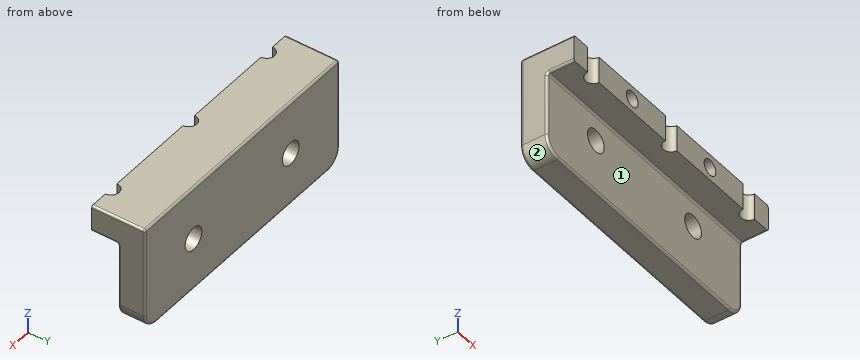
```python
from build123d import *

# Parameters (mm, degrees)
F0_W     = 50
F0_H     = 15
F1_DEPTH = 5
F2_D     = 4.3
F0_H_2   = 5
F3_DEPTH = 10
F5_D     = 2.95
F6_R     = 3
F7_R     = 0.4
F9_D     = 3
F9_DEPTH = 6
F9_TIP   = 0.9012909285


with BuildPart() as f1:
    # F0 (on Front) → F1 (new body)
    with BuildSketch(Plane.XZ):
        with Locations((0, -2.5)):
            Rectangle(F0_W, F0_H)
    extrude(amount=F1_DEPTH)

    # F2 (through all)
    with Locations(Plane(origin=(0, 0, 0), x_dir=(1, 0, 0), z_dir=(0, 1, 0))):
        with Locations((12.5, 0), (-12.5, 0)):
            Hole(F2_D / 2)

    # F0 (on Front) → F3 (join)
    with BuildSketch(Plane.XZ):
        with Locations((0, 7.5)):
            Rectangle(F0_W, F0_H_2)
    extrude(amount=F3_DEPTH)

    # F5 (through all)
    with Locations(Plane.XY.offset(10)):
        with Locations((-20, -10), (0, -10), (20, -10)):
            Hole(F5_D / 2)

    # F6
    f6_edges = [f1.edges().sort_by_distance(p)[0] for p in [
        (-25, -2.5, -10),
        (25, -2.5, -10),
    ]]
    fillet(f6_edges, radius=F6_R)

    # F7
    f7_edges = [f1.edges().sort_by_distance(p)[0] for p in [
        (0, 0, 10),
        (-25, 0, 1.5),
        (-25, -5, 10),
        (25, -5, 10),
        (0, -5, -10),
        (0, -5, 5),
        (25, -5, -1),
        (25, -7.5, 5),
        (25, 0, 1.5),
        (24.12132, -5, -9.12132),
        (-25, -5, -1),
        (-24.12132, -5, -9.12132),
        (24.12132, 0, -9.12132),
        (-25, -7.5, 5),
        (0, 0, -10),
        (-24.12132, 0, -9.12132),
    ]]
    fillet(f7_edges, radius=F7_R)

    # F9
    with Locations(Plane.XZ.offset(10)):
        with Locations((-10, 7.5), (10, 7.4705528095)):
            Hole(F9_D / 2, depth=F9_DEPTH)
            with Locations((0, 0, -(F9_DEPTH + F9_TIP / 2))):  # 118° drill point
                Cone(0, F9_D / 2, F9_TIP, mode=Mode.SUBTRACT)


solid = f1.part
```
Verification items for the finished model (mm, model axes). Face numbers are marked on the shaded views. A direction names the side the tool comes from. Coordinates: 2 decimals unless noted, no trailing zeros. Write each loop counter-clockwise with the first axis right and the second up, starting at its lowest first coordinate (ties: lowest second). Pieces come first, ordered by that corner, then holes. Notation, with made-up numbers: M 65,75.25 L 76,75.25 A30 ccw 76,105.25 Z; hole C 6,16.25 d9. An arc over 180 degrees is marked long. Answer as a JSON object with one key per item and string values. Group by question number.
(1) Cross-section at C-C, the plane y = -9.5. Record the cut outline in (x, z).
(2) Material ranges on line 1 (X direction, y = -6.4, z = 7.5); line 2 (Z direction, x = 10, y = -7.95); line 3 (Z direction, x = -12.5, y = -0.95), recorded low to high.
(3) Cross-section at D-D, the plane x = 0. Record the cut outline in (y, z) (3 decimals).
(4) Cross-section at B-B, the plane z = 0. Record the cut outline in (x, y), and give its area (3 significant figures).
(5) Tool access check on the marked faces 1 and 2. Record the directions out of +Z, -Z, +X, -X, +Y, -Y that give a thin tool (end or side, any length) a straight path to the whole face; none if there is none.
(6) Gauge pin test, flat ends, axial feed: pin 1 (3.5 mm diameter, centred on x = 12.5, z = 0, fed in from +Y) (1 decimal); pin 2 (5 mm diameter, centred on x = -1, y = -7, fed in from -Z). Record the tip position at first contact, or that the pin passes through.
(7) Cross-section at A-A, the plane x = 12.5. Record the cut outline in (y, z).
Reply:
{
 "1": {"outline": "M -25,5.4 A0.4 ccw -24.6,5 L -21.39,5 L -21.39,10 L -24.6,10 A0.4 ccw -25,9.6 Z; M -18.61,5 L -1.39,5 L -1.39,10 L -18.61,10 Z; M 1.39,5 L 18.61,5 L 18.61,10 L 1.39,10 Z; M 21.39,5 L 24.6,5 A0.4 ccw 25,5.4 L 25,9.6 A0.4 ccw 24.6,10 L 21.39,10 Z; hole C -10,7.5 d3; hole C 10,7.47 d3"},
 "2": {"line 1": "-25 to -11.5, -8.5 to 8.5, 11.5 to 25", "line 2": "5 to 5.97, 8.97 to 10", "line 3": "-10 to -2.15, 2.15 to 10"},
 "3": {"outline": "M -8.525,5 L -5.4,5 A0.4 cw -5,4.6 L -5,-9.6 A0.4 ccw -4.6,-10 L -0.4,-10 A0.4 ccw 0,-9.6 L 0,9.6 A0.4 ccw -0.4,10 L -8.525,10 Z"},
 "4": {"outline": "M -25,-4.6 A0.4 ccw -24.6,-5 L -14.65,-5 L -14.65,0 L -24.6,0 A0.4 ccw -25,-0.4 Z; M -10.35,-5 L 10.35,-5 L 10.35,0 L -10.35,0 Z; M 14.65,-5 L 24.6,-5 A0.4 ccw 25,-4.6 L 25,-0.4 A0.4 ccw 24.6,0 L 14.65,0 Z", "area": "207 mm²"},
 "5": {"face 1": "-Z, +X, -X, -Y", "face 2": "-Z, -X, +Y, -Y"},
 "6": {"pin 1": "through", "pin 2": "z = -10"},
 "7": {"outline": "M -10,5 L -5.4,5 A0.4 cw -5,4.6 L -5,2.15 L 0,2.15 L 0,9.6 A0.4 ccw -0.4,10 L -10,10 Z; M -5,-9.6 A0.4 ccw -4.6,-10 L -0.4,-10 A0.4 ccw 0,-9.6 L 0,-2.15 L -5,-2.15 Z"}
}
